Read the model definition and answer for the solid it produces. Units are mm, in the model's axes. Face numbers are marked on the shaded views. A direction names the side the tool comes from. Coordinates: 2 decimals unless noted, no trailing zeros. Use a Markdown table: item, result.
from build123d import *

# Parameters (mm, degrees)
SKETCH1_W           = 560
SKETCH1_H           = 400
BOSS_EXTRUDE1_DEPTH = 419.1
SKETCH2_W           = 509.762265323
SKETCH2_H           = 294.60835285
SKETCH2_W_2         = 160.630106896
SKETCH2_H_2         = 328.11637689
CUT_EXTRUDE1_DEPTH  = 0.0254
CUT_EXTRUDE2_START  = -60.96
SKETCH3_W           = 758.952
SKETCH3_H           = 400
SKETCH3_W_2         = 745.362874068
SKETCH3_H_2         = 373.171162969
CUT_EXTRUDE2_DEPTH  = 5.08
SKETCH5_W           = 30.340291286
SKETCH5_H           = 28.006422725
SKETCH5_W_2         = 142.365982185
SKETCH5_H_2         = 49.011239769
BOSS_EXTRUDE3_DEPTH = 2.54
SKETCH6_W           = 1.719763346
SKETCH6_H           = 400
CUT_EXTRUDE3_DEPTH  = 63.5


with BuildPart() as part:
    # Sketch1 → Boss-Extrude1 (new body)
    with BuildSketch(Plane.XY):
        with Locations((161.193919926, -4.872504675)):
            Rectangle(SKETCH1_W, SKETCH1_H)
    extrude(amount=BOSS_EXTRUDE1_DEPTH)

    # Sketch2 → Cut-Extrude1 (cut)
    with BuildSketch(Plane.XY.offset(419.1)):
        with Locations((-19.802766229, -4.093923129)):
            Rectangle(SKETCH2_W, SKETCH2_H)
        with Locations((339.761572352, -22.10119724)):
            Rectangle(SKETCH2_W_2, SKETCH2_H_2)
    extrude(amount=-CUT_EXTRUDE1_DEPTH, mode=Mode.SUBTRACT)

    # Sketch3 → Cut-Extrude2 (cut)
    with BuildSketch(Plane.XY.offset(419.1).offset(CUT_EXTRUDE2_START)):
        with Locations((61.717919926, -4.872504675)):
            Rectangle(SKETCH3_W, SKETCH3_H)
        with Locations((61.107514964, -10.347774784)):
            Rectangle(SKETCH3_W_2, SKETCH3_H_2, mode=Mode.SUBTRACT)
    extrude(amount=-CUT_EXTRUDE2_DEPTH, mode=Mode.SUBTRACT)

    # Sketch5 → Boss-Extrude3 (add)
    with BuildSketch(Plane.XY.offset(419.0746)):
        with Locations((321.924411259, 55.397530231)):
            Rectangle(SKETCH5_W, SKETCH5_H)
        with Locations((339.837256709, 102.463879533)):
            Rectangle(SKETCH5_W_2, SKETCH5_H_2)
        with Locations((283.824411259, 55.397530231)):
            Rectangle(SKETCH5_W, SKETCH5_H)
        with Locations((360.024411259, 55.397530231)):
            Rectangle(SKETCH5_W, SKETCH5_H)
        with Locations((398.124411259, 55.397530231)):
            Rectangle(SKETCH5_W, SKETCH5_H)
        with Locations((321.924411259, 22.377530231)):
            Rectangle(SKETCH5_W, SKETCH5_H)
        with Locations((360.024411259, 22.377530231)):
            Rectangle(SKETCH5_W, SKETCH5_H)
        with Locations((398.124411259, 22.377530231)):
            Rectangle(SKETCH5_W, SKETCH5_H)
        with Locations((321.924411259, -10.642469769)):
            Rectangle(SKETCH5_W, SKETCH5_H)
        with Locations((360.024411259, -10.642469769)):
            Rectangle(SKETCH5_W, SKETCH5_H)
        with Locations((398.124411259, -10.642469769)):
            Rectangle(SKETCH5_W, SKETCH5_H)
        with Locations((321.924411259, -43.66246977)):
            Rectangle(SKETCH5_W, SKETCH5_H)
        with Locations((360.024411259, -43.66246977)):
            Rectangle(SKETCH5_W, SKETCH5_H)
        with Locations((398.124411259, -43.66246977)):
            Rectangle(SKETCH5_W, SKETCH5_H)
        with Locations((321.924411259, -76.68246977)):
            Rectangle(SKETCH5_W, SKETCH5_H)
        with Locations((360.024411259, -76.68246977)):
            Rectangle(SKETCH5_W, SKETCH5_H)
        with Locations((398.124411259, -76.68246977)):
            Rectangle(SKETCH5_W, SKETCH5_H)
        with Locations((321.924411259, -109.702469769)):
            Rectangle(SKETCH5_W, SKETCH5_H)
        with Locations((360.024411259, -109.702469769)):
            Rectangle(SKETCH5_W, SKETCH5_H)
        with Locations((398.124411259, -109.702469769)):
            Rectangle(SKETCH5_W, SKETCH5_H)
        with Locations((321.924411259, -142.72246977)):
            Rectangle(SKETCH5_W, SKETCH5_H)
        with Locations((360.024411259, -142.72246977)):
            Rectangle(SKETCH5_W, SKETCH5_H)
        with Locations((398.124411259, -142.72246977)):
            Rectangle(SKETCH5_W, SKETCH5_H)
        with Locations((283.824411259, 22.377530231)):
            Rectangle(SKETCH5_W, SKETCH5_H)
        with Locations((283.824411259, -10.642469769)):
            Rectangle(SKETCH5_W, SKETCH5_H)
        with Locations((283.824411259, -43.66246977)):
            Rectangle(SKETCH5_W, SKETCH5_H)
        with Locations((283.824411259, -76.68246977)):
            Rectangle(SKETCH5_W, SKETCH5_H)
        with Locations((283.824411259, -109.702469769)):
            Rectangle(SKETCH5_W, SKETCH5_H)
        with Locations((283.824411259, -142.72246977)):
            Rectangle(SKETCH5_W, SKETCH5_H)
    extrude(amount=BOSS_EXTRUDE3_DEPTH)

    # Sketch6 → Cut-Extrude3 (cut)
    with BuildSketch(Plane.XY.offset(419.1)):
        with Locations((245.729481122, -4.872504675)):
            Rectangle(SKETCH6_W, SKETCH6_H)
    extrude(amount=-CUT_EXTRUDE3_DEPTH, mode=Mode.SUBTRACT)


solid = part.part
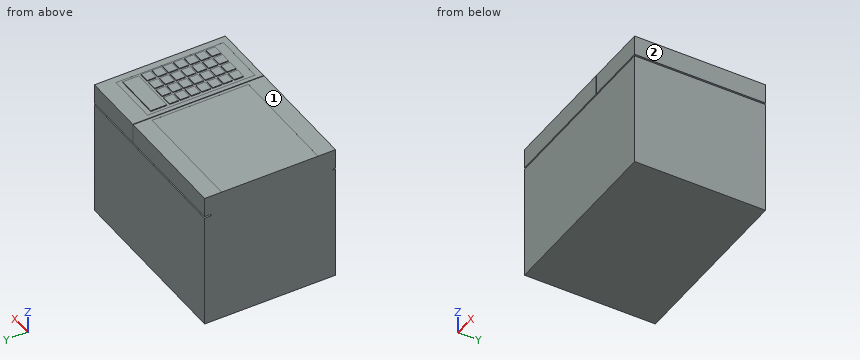
(1) For the marked faces 1 and 2, determine the directions among +Z, -Z, +X, -X, +Y, -Y from which every point of the face is accessible in a straight line to the end or side of a thin tool.
Report:
| item | result |
|---|---|
| face 1 | +Z, -X, +Y, -Y |
| face 2 | +Z, -Z, +X, +Y, -Y |
(2) Straight lines are drawn through the part: L1, parallel to Z at x = 258.5, y = -66; L2, parallel to X at y = 113, z = 367. For each, find the intervals that lie inside material, in ascending order.
Report:
| item | result |
|---|---|
| L1 | z = 0 to 419.1 |
| L2 | x = -118.81 to 244.87, 246.59 to 441.19 |
(3) Each of these flat-tipped pins is pushed along its axis until it touches: P1, Ø0.8, axis at y = 21.5, z = 420.5, coming from the -X side; P2, Ø0.8, axis at x = 279, z = 420.5, coming from the -Y side; P3, Ø10, axis at x = 92.5, y = 123, coming from the +Z side. Where does it stop, or does it pass through?
Report:
| item | result |
|---|---|
| P1 | stops at x = 268.65 |
| P2 | stops at y = -156.73 |
| P3 | stops at z = 419.07 |
